from build123d import *

# Parameters (mm, degrees)
SKETCH_1_R               = 1.5
EXTRUDE_1_DEPTH          = 4
FILLET_1_R               = 2
FILLET_2_R               = 4
SKETCH_2_R               = 1.5
EXTRUDE_2_DEPTH          = 7
CUT_EXTRUDE_1_DEPTH      = 75.524894896
CUT_EXTRUDE_1_DEPTH_BACK = 75.524894896
CUT_EXTRUDE_2_DEPTH      = 2
FILLET_3_R               = 1


with BuildPart() as part:
    # 草图1 → 凸台-拉伸1 (new, symmetric)
    with BuildSketch(Plane(origin=(0, 0, 0), x_dir=(0, 0, -1), z_dir=(1, 0, 0))):
        with BuildLine():
            Line((-59.734284448, 46.23253896), (-60.904491974, 28.270617728))
            ThreePointArc((-60.904491974, 28.270617728), (-61.260668779, 26.862087023), (-62.096445312, 25.67368547))
            Line((-62.096445312, 25.67368547), (-72.42215962, 15.555403796))
            Line((-72.42215962, 15.555403796), (-73.072274912, 5.576558667))
            Line((-73.072274912, 5.576558667), (-79.059581989, 5.966627842))
            Line((-79.059581989, 5.966627842), (-78.025468729, 21.839590984))
            Line((-78.025468729, 21.839590984), (-67.433323191, 47.994063888))
            ThreePointArc((-67.433323191, 47.994063888), (-62.833683596, 50.391827077), (-59.734284448, 46.23253896))
        make_face()
        with Locations((-64.896030026, 28.530663844)):
            Circle(SKETCH_1_R, mode=Mode.SUBTRACT)
        with Locations((-63.7258225, 46.492585076)):
            Circle(SKETCH_1_R, mode=Mode.SUBTRACT)
    extrude(amount=EXTRUDE_1_DEPTH, both=True)

    # 圆角1
    fillet_1_edges = [part.edges().sort_by_distance(p)[0] for p in [
        (0, 5.576558667, 73.072274912),
        (0, 5.966627842, 79.059581989),
    ]]
    fillet(fillet_1_edges, radius=FILLET_1_R)

    # 圆角2
    fillet_2_edges = [part.edges().sort_by_distance(p)[0] for p in [
        (0, 15.555403796, 72.42215962),
    ]]
    fillet(fillet_2_edges, radius=FILLET_2_R)

    # 草图2 → 凸台-拉伸2 (add, symmetric)
    with BuildSketch(Plane(origin=(0, 0, 0), x_dir=(0, 0, -1), z_dir=(1, 0, 0))):
        with BuildLine():
            Line((-60.534478137, 33.950088462), (-59.734284448, 46.23253896))
            ThreePointArc((-59.734284448, 46.23253896), (-62.833683596, 50.391827077), (-67.433323191, 47.994063888))
            Line((-67.433323191, 47.994063888), (-78.025468729, 21.839590984))
            Line((-78.025468729, 21.839590984), (-78.075072521, 21.07820517))
            Line((-78.075072521, 21.07820517), (-60.534478137, 33.950088462))
        make_face()
        with Locations((-63.7258225, 46.492585076)):
            Circle(SKETCH_2_R, mode=Mode.SUBTRACT)
    extrude(amount=EXTRUDE_2_DEPTH, both=True)

    # 草图3 → 切除-拉伸1 (cut, two sides: drawn at the far end of the back side and taken through both)
    with BuildSketch(Plane(origin=(0, 76.493888819, 81.941089709), x_dir=(-1, 0, 0), z_dir=(0, -0.5916260801069638, 0.8062124914296904)).offset(-CUT_EXTRUDE_1_DEPTH_BACK)):
        with BuildLine():
            Line((4, 38.964052974), (4, 30.964052974))
            Line((4, 30.964052974), (-4, 30.964052974))
            Line((-4, 30.964052974), (-4, 38.964052974))
            ThreePointArc((-4, 38.964052974), (0, 42.964052974), (4, 38.964052974))
        make_face()
        with BuildLine():
            Line((7, 38.964052974), (7, 53.964052974))
            Line((7, 53.964052974), (4, 53.964052974))
            Line((4, 53.964052974), (4, 44.70861562))
            ThreePointArc((4, 44.70861562), (6.204836823, 42.204423323), (7, 38.964052974))
        make_face()
        with BuildLine():
            Line((-4, 53.964052974), (-4, 44.70861562))
            ThreePointArc((-4, 44.70861562), (-6.204836823, 42.204423323), (-7, 38.964052974))
            Line((-7, 38.964052974), (-7, 53.964052974))
            Line((-7, 53.964052974), (-4, 53.964052974))
        make_face()
    extrude(amount=CUT_EXTRUDE_1_DEPTH + CUT_EXTRUDE_1_DEPTH_BACK, mode=Mode.SUBTRACT)

    # 草图4 → 切除-拉伸2 (cut, symmetric)
    with BuildSketch(Plane(origin=(0, 0, 0), x_dir=(0, 0, -1), z_dir=(1, 0, 0))):
        with BuildLine():
            Line((-68.896030026, 28.530663844), (-68.896030026, 30.611669816))
            Line((-68.896030026, 30.611669816), (-72.22581768, 28.168158659))
            Line((-72.22581768, 28.168158659), (-75.063263573, 21.161844268))
            Line((-75.063263573, 21.161844268), (-76.06592845, 5.771593254))
            Line((-76.06592845, 5.771593254), (-75.068043938, 5.706581725))
            ThreePointArc((-75.068043938, 5.706581725), (-73.618739254, 6.199188753), (-72.942251853, 7.572327692))
            Line((-72.942251853, 7.572327692), (-72.52160152, 14.029035582))
            ThreePointArc((-72.52160152, 14.029035582), (-72.165424714, 15.437566287), (-71.329648181, 16.62596784))
            Line((-71.329648181, 16.62596784), (-62.096445312, 25.67368547))
            ThreePointArc((-62.096445312, 25.67368547), (-66.445491407, 24.842958673), (-68.896030026, 28.530663844))
        make_face()
    extrude(amount=CUT_EXTRUDE_2_DEPTH, both=True, mode=Mode.SUBTRACT)

    # 圆角3
    fillet_3_edges = [part.edges().sort_by_distance(p)[0] for p in [
        (0, 28.168158659, 72.22581768),
        (0, 30.611669816, 68.896030026),
        (0, 5.771593254, 76.06592845),
        (0, 21.161844268, 75.063263573),
    ]]
    fillet(fillet_3_edges, radius=FILLET_3_R - 0.0001)  # a hair under: the kernel refuses the full size


solid = part.part
The listing builds one solid part. Answer for the finished solid, in the listing's coordinates (mm). A direction names the side the tool comes from. Coordinates: 2 decimals unless noted, no trailing zeros. Write each loop counter-clockwise with the first axis right and the second up, starting at its lowest first coordinate (ties: lowest second). Pieces come first, ordered by that corner, then holes. Notation, with made-up numbers: (36.25, 51) - (88.25, 51) arc R18 cw to (88.25, 56) - close; hole circle Ø5 at (48.25, 23.5). An arc over 180 degrees is marked (long way). Return JSON: item names as keys, results as strings.
1. For a pull along Z with two mould halves and no side action, classify faces 4 (the face through (2.72, 5.77, 76.05)), 5 (the face through (4, 20, 72)), 6 (the face through (0.03, 28.9, 71.23)) as +Z half, -Z half, draft (parallel to the pull), parting line (faces both ways), or undercut.
Final values:
{"face 4": "+Z half", "face 5": "draft", "face 6": "undercut"}
2. Which of the six approach directions +Z, -Z, +X, -X, +Y, -Y give full straight-line access (tool end or side, diameter ignored) to faces 1 (the face through (2, 19, 71)), 2 (the face through (0.03, 13.98, 75.53)), 3 (the face through (-4, 44, 66))?
Final values:
{"face 1": "-Y", "face 2": "-Z, -Y", "face 3": "+Z, +Y"}
3. The part is cut by section C-C on z = 64.25. Count the separate pieces of the cut face and the enclosed holes in it, then the cut area to 3 significant figures.
Final values:
{"separate pieces": "4", "enclosed holes": "0", "area": "153 mm^2"}
4. Each of these flat-tipped pins is pushed along its axis until it touches: pin 1 Ø6 at (x, y) = (-4.5, 36.5) entering from +Z; pin 2 Ø7.5 at (y, z) = (17, 71) entering from +X; pin 3 Ø8 at (x, z) = (2.5, 65) entering from -Y; pin 4 Ø1.8 at (y, z) = (28.53, 64.9) entering from -X. Where does it stop, or does it pass through?
Final values:
{"pin 1": "z = 73.3", "pin 2": "x = 4", "pin 3": "y = 18.91", "pin 4": "through"}
5. The part is cut by section A-A on x = -3.5. Determine the outline of the cut face in (y, z), then the cut area to 3 significant figures.
Final values:
{"outline": "(5.71, 75.07) arc R2 ccw to (7.57, 72.94) - (14.03, 72.52) arc R4 cw to (16.63, 71.33) - (25.67, 62.1) arc R4 ccw to (28.27, 60.9) - (41.85, 60.02) - (31.51, 74.11) - (21.84, 78.03) - (7.96, 78.93) arc R2 ccw to (5.84, 77.06) - close; hole circle Ø3 at (28.53, 64.9)", "area": "310 mm^2"}
6. The part is cut by section B-B on y = 11. Determine the outline of the cut face in (x, z), then the cut area to 3 significant figures.
Final values:
{"outline": "(-4, 72.72) - (-2, 72.72) - (-2, 75.73) - (2, 75.73) - (2, 72.72) - (4, 72.72) - (4, 78.73) - (-4, 78.73) - close", "area": "36.1 mm^2"}
7. Consider line 1 along X through (y, z) = (21, 69.75); line 2 along X through (y, z) = (48, 66); line 3 along X through (y, z) = (27, 67.75). Determine where each line is inside the solid, lowest interval first.
Final values:
{"line 1": "-4 to -2, 2 to 4", "line 2": "-7 to -4, 4 to 7", "line 3": "-4 to 4"}
